from build123d import *

# Parameters (mm, degrees)
F0_W     = 60
F0_H     = 35
F1_DEPTH = 20
F3_DEPTH = 25


# Not quite as in the source:
# - a feature names something its author has since deleted; it is built from what else it names


with BuildPart() as f1:
    # F0 (on Front) → F1 (new body)
    with BuildSketch(Plane.XZ):
        with Locations((30, 17.5)):
            Rectangle(F0_W, F0_H)
    extrude(amount=F1_DEPTH)

    # F2 (on face) → F3 (cut)
    with BuildSketch(Plane.XZ.offset(20)):
        Polygon((60, 35), (30, 35), (60, 17.5), align=None)
    extrude(amount=-F3_DEPTH, mode=Mode.SUBTRACT)


solid = f1.part
Can you work these out from the model? Positions are in its coordinate system, mm. Coordinates: 2 decimals unless noted, no trailing zeros. Order: outer loops, then holes, each group sorted by start corner. A loop starts at its lowest first (then second) coordinate and runs counter-clockwise, first axis right, second up. Notation, with made-up numbers: (-5.5, 52.5) -> (15.5, 52.5) arc R14 ccw to (15.5, 67.5) -> close; hole circle Ø6 at (-9, 57). An arc over 180 degrees is marked (long way). Use one line per item in the form item = value.
Q1. I need wall thicknesses on L1, parallel to X at y = -5, z = 22.5; L2, parallel to Z at x = 41.5, y = -17.5; L3, parallel to Z at x = 46, y = -13.5. Which ranges of each line are inside material? Lowest first, please.
From the geometry:
L1 = 0 to 51.43
L2 = 0 to 28.29
L3 = 0 to 25.67
Q2. Will these pins go through, and if not, where does the flat tip stop? P1, Ø6, axis at y = -17, z = 15.5, coming from the -X side; P2, Ø4, axis at x = 53.5, y = -7.5, coming from the +Z side; P3, Ø3, axis at y = -9.5, z = 22, coming from the +X side.
From the geometry:
P1 = 0
P2 = 22.46
P3 = 54.86
Q3. Imagine slicing it at B-B, the plane z = 30.5. List the corners of the cut face in (x, y) for me, then the cut area to 3 significant figures.
From the geometry:
outline = (0, -20) -> (37.71, -20) -> (37.71, 0) -> (0, 0) -> close
area = 754 mm²
Q4. Imagine slicing it at C-C, the plane x = 42. List the corners of the cut face in (y, z) for me.
From the geometry:
outline = (-20, 0) -> (0, 0) -> (0, 28) -> (-20, 28) -> close
Q5. Imagine slicing it at A-A, the plane y = -13.25. List the corners of the cut face in (x, z) for me.
From the geometry:
outline = (0, 0) -> (60, 0) -> (60, 17.5) -> (30, 35) -> (0, 35) -> close
